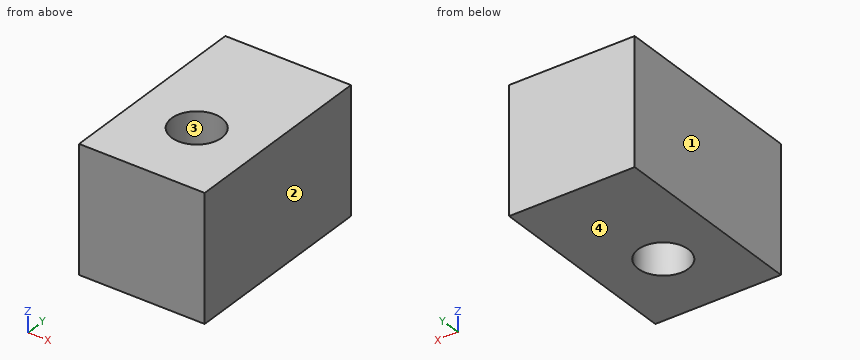
```python
from build123d import *

# Parameters (mm, degrees)
SKETCH1_W           = 10
SKETCH1_H           = 16
SKETCH1_R           = 2
BOSS_EXTRUDE1_DEPTH = 10


with BuildPart() as part:
    # Sketch1 → Boss-Extrude1 (new body)
    with BuildSketch(Plane(origin=(0, 0, 0), x_dir=(-1.0, 0, 8.723016310561762e-12), z_dir=(-8.723016310561762e-12, 5.3094256425393756e-15, -1.0))):
        with Locations((79.539990831, 54.5)):
            Rectangle(SKETCH1_W, SKETCH1_H)
        with Locations((79.539990831, 52.5)):
            Circle(SKETCH1_R, mode=Mode.SUBTRACT)
    extrude(amount=-BOSS_EXTRUDE1_DEPTH)


solid = part.part
```
Design review of the part built by this model. Coordinates are the model's own, in mm. Face numbers are marked on the shaded views. Coordinates: 2 decimals unless noted, no trailing zeros. Order: outer loops, then holes, each group sorted by start corner. A loop starts at its lowest first (then second) coordinate and runs counter-clockwise, first axis right, second up.
1) Mouldability with a two-part tool opening along X and no side actions: class the marked faces 1, 2, 3 and 4 as +X half, -X half, draft (parallel to the pull), parting line (faces both ways), or undercut.
2) Take a section at C-C, the plane x = -79.25. Give the boundary of the cut face in (y, z).
3) Take a section at B-B, the plane z = 3.5. Give the boundary of the cut face in (x, y).
4) Clearance check with a flat-ended pin moving along its axis: pin 1 (4.5 mm diameter, centred on x = -79.54, y = 52.5, fed in from -Z). State where the tip first meets the part, or that it passes through.
5) Wall thickness on line 1 along X through (y, z) = (52.5, 2); line 2 along Y through (x, z) = (-78.25, 3.25); line 3 along Y through (x, z) = (-80, 6.5): over which ranges is each line inside the solid? List them lowest first.
6) Take a section at A-A, the plane y = 52.5. Give the boundary of the cut face in (x, z), and give its area (3 significant figures).
Returned:
1. face 1: -X half
1. face 2: +X half
1. face 3: undercut
1. face 4: draft
2. outline: (46.5, 0) - (50.52, 0) - (50.52, 10) - (46.5, 10) - close; (54.48, 0) - (62.5, 0) - (62.5, 10) - (54.48, 10) - close
3. outline: (-84.54, 46.5) - (-74.54, 46.5) - (-74.54, 62.5) - (-84.54, 62.5) - close; hole circle Ø4 at (-79.54, 52.5)
4. pin 1: stops at z = 0
5. line 1: x = -84.54 to -81.54, -77.54 to -74.54
5. line 2: y = 46.5 to 50.97, 54.03 to 62.5
5. line 3: y = 46.5 to 50.55, 54.45 to 62.5
6. outline: (-84.54, 0) - (-81.54, 0) - (-81.54, 10) - (-84.54, 10) - close; (-77.54, 0) - (-74.54, 0) - (-74.54, 10) - (-77.54, 10) - close
6. area: 60.0 mm2
